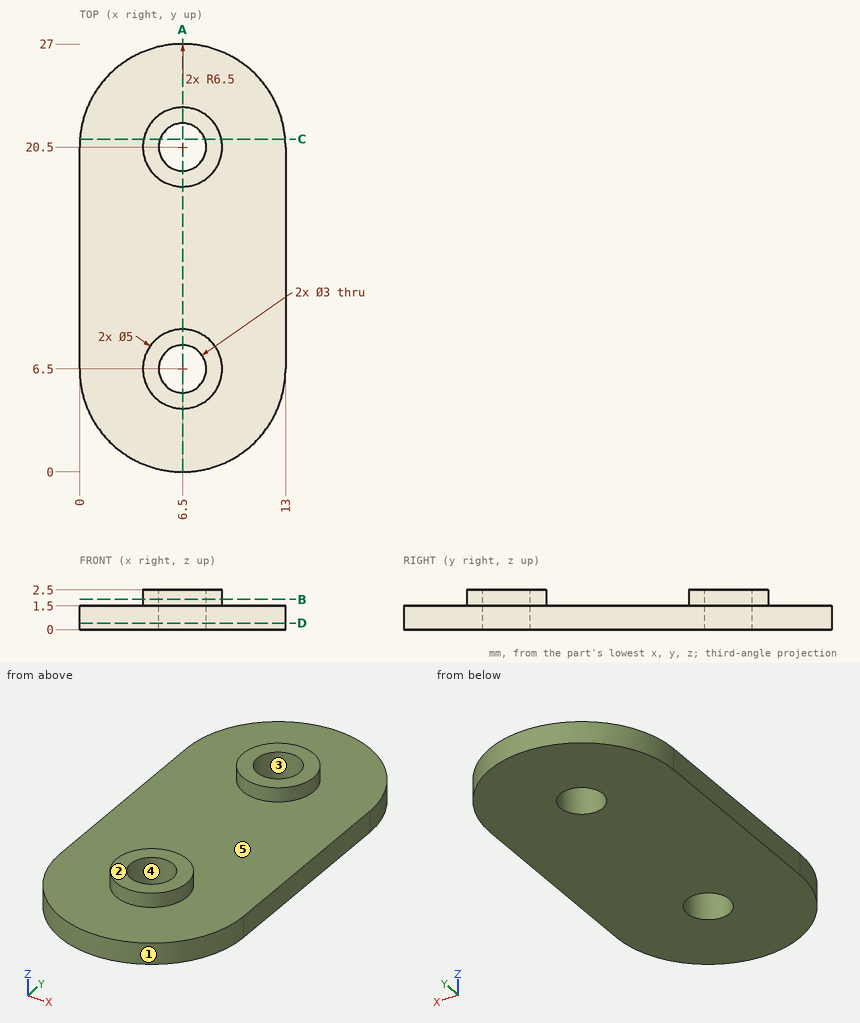
Check sheet for the drawn part. Datum: minimum x, y, z corner. Units: mm. A direction names the side the tool comes from. Give positions to 0.01 mm unless a question says otherwise; leave off trailing zeros. Order: outer loops, then holes, each group sorted by start corner. A loop starts at its lowest first (then second) coordinate and runs counter-clockwise, first axis right, second up. Notation, with made-up numbers: (61, 87) - (105, 87) arc R22 cw to (105, 118) - close; hole circle Ø5 at (59.5, 82). An arc over 180 degrees is marked (long way). Answer as a JSON object with one key per item and string values.
(1) Tool access check on the marked faces 4 and 5. Record the directions out of +Z, -Z, +X, -X, +Y, -Y that give a thin tool (end or side, any length) a straight path to the whole face; none if there is none.
Report:
{"face 4": "+Z, -Z", "face 5": "+Z"}
(2) Cross-section at B-B (z = 1.9). Record the cut outline in (x, y), then the cut area to 3 significant figures.
Report:
{"outline": "circle Ø5 at (6.5, 6.5); circle Ø5 at (6.5, 20.5); hole circle Ø3 at (6.5, 6.5); hole circle Ø3 at (6.5, 20.5)", "area": "25.1 mm^2"}
(3) Material ranges on line 1 (Y direction, x = 6.5, z = 1); line 2 (Y direction, x = 6.5, z = 1.55); line 3 (X direction, y = 20.5, z = 0.85), recorded low to high.
Report:
{"line 1": "0 to 5, 8 to 19, 22 to 27", "line 2": "4 to 5, 8 to 9, 18 to 19, 22 to 23", "line 3": "0 to 5, 8 to 13"}
(4) Draft check along Y on the marked faces 1, 2 and 3. Enter one of: released by +Y, released by -Y, zero draft, split by the parting line, or undercut.
Report:
{"face 1": "released by -Y", "face 2": "zero draft", "face 3": "undercut"}
(5) Cross-section at D-D (z = 0.4). Record the cut outline in (x, y), then the cut area to 3 significant figures.
Report:
{"outline": "(0, 6.5) arc R6.5 ccw to (13, 6.5) - (13, 20.5) arc R6.5 ccw to (0, 20.5) - close; hole circle Ø3 at (6.5, 6.5); hole circle Ø3 at (6.5, 20.5)", "area": "301 mm^2"}
(6) Cross-section at C-C (y = 21). Record the cut outline in (x, z).
Report:
{"outline": "(0.02, 0) - (5.09, 0) - (5.09, 2.5) - (4.05, 2.5) - (4.05, 1.5) - (0.02, 1.5) - close; (7.91, 0) - (12.98, 0) - (12.98, 1.5) - (8.95, 1.5) - (8.95, 2.5) - (7.91, 2.5) - close"}
(7) Cross-section at A-A (x = 6.5). Record the cut outline in (y, z).
Report:
{"outline": "(0, 0) - (5, 0) - (5, 2.5) - (4, 2.5) - (4, 1.5) - (0, 1.5) - close; (8, 0) - (19, 0) - (19, 2.5) - (18, 2.5) - (18, 1.5) - (9, 1.5) - (9, 2.5) - (8, 2.5) - close; (22, 0) - (27, 0) - (27, 1.5) - (23, 1.5) - (23, 2.5) - (22, 2.5) - close"}
(8) Depth check by flat-ended pin: pin 1 Ø1.5 at (x, y) = (10, 7.5) entering from +Z; pin 2 Ø1 at (x, z) = (9, 0.5) entering from +Y. Enter the tip coordinate at first touch or a pass-through.
Report:
{"pin 1": "z = 1.5", "pin 2": "y = 26.68"}
